```python
from build123d import *

# Parameters (mm, degrees)
F1_DEPTH = 18.16
F2_W     = 12
F2_H     = 4.5
F3_DEPTH = 12
F4_R     = 5.99999


# Not quite as in the source:
# - a fillet or chamfer is up to 0.001 mm smaller than in the source, because OpenCascade refuses the exact size


with BuildPart() as f1:
    # F0 (on Top) → F1 (new body)
    with BuildSketch(Plane.XY):
        Polygon((18.16, 0), (-18.16, 0), (-18.16, -8), (-14.98, -8), (-14.98, -4), (14.98, -4), (14.98, -8), (18.16, -8), align=None)
    extrude(amount=F1_DEPTH)

    # F2 (on face) → F3 (join)
    with BuildSketch(Plane(origin=(0, 0, 0), x_dir=(1, 0, 0), z_dir=(0, 0, -1))):
        with Locations((-24.16, 5.75)):
            Rectangle(F2_W, F2_H)
        with Locations((24.16, 5.75)):
            Rectangle(F2_W, F2_H)
    extrude(amount=-F3_DEPTH)

    # F4 (radius 6 in the source; OpenCascade refuses exactly that, so slightly less here)
    f4_edges = [f1.edges().sort_by_distance(p)[0] for p in [
        (-30.16, -5.75, 12),
        (-30.16, -5.75, 0),
        (30.16, -5.75, 0),
        (30.16, -5.75, 12),
    ]]
    fillet(f4_edges, radius=F4_R)


solid = f1.part
```
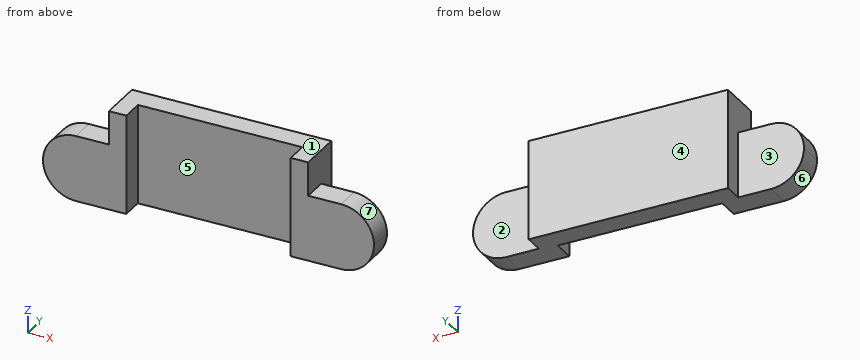
Here's how the part is built. I have some questions about the finished solid (model axes, mm). Face numbers are marked on the shaded views. A direction names the side the tool comes from. Round coordinates to 2 decimals unless told otherwise and drop trailing zeros. Loops run counter-clockwise (first coordinate to the right, second up) from the corner with the lowest first, then second, coordinate; pieces in that order, holes last. Notation, with made-up numbers: (-16.5, 65) -> (-6.5, 65) arc R13 ccw to (-6.5, 73) -> close; hole circle Ø2 at (73, -0.75). An arc over 180 degrees is marked (long way). Answer as CSV lines item,"result". Start each with the question number.
1. Imagine slicing it at D-D on y = -1. Write out the boundary of the cut face in (x, z).
2. For the marked faces 1, 2 and 3, which set-ups out of +Z, -Z, +X, -X, +Y, -Y let a thin tool reach every point of the face, with its end or its side?
3. Imagine slicing it at A-A on z = 14.75. Write out the boundary of the cut face in (x, y).
4. If we mould it in two halves opening along X, with no side actions, what happens to the marked faces 4, 5, 6 and 7? For each: pulls with the +X half, pulls with the -X half, needs draft (parallel to the pull), parting line crosses it, or undercut.
5. I'm going to push flat-ended pins straight in: P1, Ø1.5, axis at x = 1.5, z = 8.5, coming from the -Y side; P2, Ø1.2, axis at y = -6.5, z = 9, coming from the -X side; P3, Ø4, axis at y = -3, z = 9.5, coming from the -X side. Where does each tip first touch, or does it pass through?
6. Imagine slicing it at C-C on x = 2. Write out the boundary of the cut face in (y, z), plus the area to 3 significant figures.
7. I need wall thicknesses on probe 1 along X at (y, z) = (-5.25, 12.25); probe 2 along X at (y, z) = (-2.5, 6.5); probe 3 along Y at (x, z) = (24, 2.5). Which ranges of each line are inside material? Lowest first, please. Write a range as from..to.
Solution:
1,outline,"(-18.16, 0) -> (18.16, 0) -> (18.16, 18.16) -> (-18.16, 18.16) -> close"
2,face 1,"+Z, +X, -X, +Y, -Y"
2,face 2,"+Z, -Z, +X, +Y"
2,face 3,"+Z, -Z, -X, +Y"
3,outline,"(-18.16, -8) -> (-14.98, -8) -> (-14.98, -4) -> (14.98, -4) -> (14.98, -8) -> (18.16, -8) -> (18.16, 0) -> (-18.16, 0) -> close"
4,face 4,"needs draft"
4,face 5,"undercut"
4,face 6,"pulls with the -X half"
4,face 7,"pulls with the +X half"
5,P1,"y = -4"
5,P2,"x = -29.66"
5,P3,"x = -29.95"
6,outline,"(-4, 0) -> (0, 0) -> (0, 18.16) -> (-4, 18.16) -> close"
6,area,"72.6 mm²"
7,probe 1,"-18.16..-14.98, 14.98..18.16"
7,probe 2,"-18.16..18.16"
7,probe 3,"-8..-3.5"
